```python
from build123d import *

# Parameters (mm, degrees)
SKETCH_1_R               = 6
EXTRUDE_1_DEPTH          = 15
SKETCH_2_OUTSIDE_W       = 18.53
SKETCH_2_OUTSIDE_H       = 18.53
SKETCH_2_OUTSIDE_W_2     = 10
SKETCH_2_OUTSIDE_H_2     = 17.562426414
CUT_EXTRUDE_1_DEPTH      = 15
EXTRUDE_2_DEPTH          = 1
SKETCH_4_W               = 10
SKETCH_4_H               = 12
EXTRUDE_3_DEPTH          = 10
SKETCH_5_R               = 1.5
EXTRUDE_4_DEPTH          = 10
SKETCH_6_W               = 6.926984356
SKETCH_6_H               = 2.009610912
CUT_EXTRUDE_2_DEPTH      = 10
SKETCH_7_R               = 5
EXTRUDE_5_DEPTH          = 4
SKETCH_8_W               = 7.4
SKETCH_8_H               = 10
EXTRUDE_6_DEPTH          = 4
HOLE_WIZARD_M1_4_1_D     = 1.6
HOLE_WIZARD_M1_4_1_DEPTH = 10
HOLE_WIZARD_M1_4_1_TIP   = 0.480688495
HOLE_WIZARD_M1_6_1_D     = 1.25
HOLE_WIZARD_M1_6_1_DEPTH = 4
HOLE_WIZARD_M1_6_1_TIP   = 0.375537887


with BuildPart() as part:
    # 草图1 → 凸台-拉伸1 (new body)
    with BuildSketch(Plane(origin=(0, 0, 0), x_dir=(1, 0, 0), z_dir=(0, 1, 0))):
        with Locations(Location((0, 0, 0), (0, 0, 270))):
            Circle(SKETCH_1_R)
    extrude(amount=EXTRUDE_1_DEPTH)

    # 草图2 outside → 切除-拉伸1 (cut)
    with BuildSketch(Plane(origin=(0, 15, 0), x_dir=(1, 0, 0), z_dir=(0, 1, 0))):
        Rectangle(SKETCH_2_OUTSIDE_W, SKETCH_2_OUTSIDE_H)
        Rectangle(SKETCH_2_OUTSIDE_W_2, SKETCH_2_OUTSIDE_H_2, mode=Mode.SUBTRACT)
    extrude(amount=-CUT_EXTRUDE_1_DEPTH, mode=Mode.SUBTRACT)

    # 草图3 → 凸台-拉伸2 (add)
    with BuildSketch(Plane(origin=(0, 15, 0), x_dir=(1, 0, 0), z_dir=(0, 1, 0))):
        with BuildLine():
            Line((0, -6), (-15, -6))
            Line((-15, -6), (-15, 6))
            Line((-15, 6), (0, 6))
            ThreePointArc((0, 6), (2.837274331, 5.286764074), (5, 3.31662479))
            Line((5, 3.31662479), (5, -3.31662479))
            ThreePointArc((5, -3.31662479), (2.837274331, -5.286764074), (0, -6))
        make_face()
    extrude(amount=EXTRUDE_2_DEPTH)

    # 草图4 → 凸台-拉伸3 (add)
    with BuildSketch(Plane.XZ):
        Rectangle(SKETCH_4_W, SKETCH_4_H)
    extrude(amount=EXTRUDE_3_DEPTH)

    # 草图5 → 凸台-拉伸4 (add)
    with BuildSketch(Plane.XZ.offset(10)):
        with Locations(Location((0, 0, 0), (0, 0, 270))):
            Circle(SKETCH_5_R)
    extrude(amount=EXTRUDE_4_DEPTH)

    # 草图6 → 切除-拉伸2 (cut)
    with BuildSketch(Plane.XZ.offset(20)):
        with Locations((0.466792476, -2.004805456)):
            Rectangle(SKETCH_6_W, SKETCH_6_H)
    extrude(amount=-CUT_EXTRUDE_2_DEPTH, mode=Mode.SUBTRACT)

    # 草图7 → 凸台-拉伸5 (add)
    with BuildSketch(Plane(origin=(0, 16, 0), x_dir=(1, 0, 0), z_dir=(0, 1, 0))):
        Circle(SKETCH_7_R)
    extrude(amount=EXTRUDE_5_DEPTH)

    # 草图8 → 凸台-拉伸6 (add)
    with BuildSketch(Plane(origin=(0, 16, 0), x_dir=(1, 0, 0), z_dir=(0, 1, 0))):
        with Locations((-13.7, 0)):
            Rectangle(SKETCH_8_W, SKETCH_8_H)
    extrude(amount=EXTRUDE_6_DEPTH)

    # M1.4 间隙孔1
    with Locations(Plane(origin=(0, -10, 0), x_dir=(-1, 0, 0), z_dir=(0, -1, 0))):
        with Locations((-2.5, 3.75), (2.5, -3.75)):
            Hole(HOLE_WIZARD_M1_4_1_D / 2, depth=HOLE_WIZARD_M1_4_1_DEPTH)
            with Locations((0, 0, -(HOLE_WIZARD_M1_4_1_DEPTH + HOLE_WIZARD_M1_4_1_TIP / 2))):  # 118° drill point
                Cone(0, HOLE_WIZARD_M1_4_1_D / 2, HOLE_WIZARD_M1_4_1_TIP, mode=Mode.SUBTRACT)

    # M1.6 螺纹孔1
    with Locations(Plane(origin=(0, -10, 0), x_dir=(-1, 0, 0), z_dir=(0, -1, 0))):
        with Locations((0, 5), (0, -5)):
            Hole(HOLE_WIZARD_M1_6_1_D / 2, depth=HOLE_WIZARD_M1_6_1_DEPTH)
            with Locations((0, 0, -(HOLE_WIZARD_M1_6_1_DEPTH + HOLE_WIZARD_M1_6_1_TIP / 2))):  # 118° drill point
                Cone(0, HOLE_WIZARD_M1_6_1_D / 2, HOLE_WIZARD_M1_6_1_TIP, mode=Mode.SUBTRACT)


solid = part.part
```
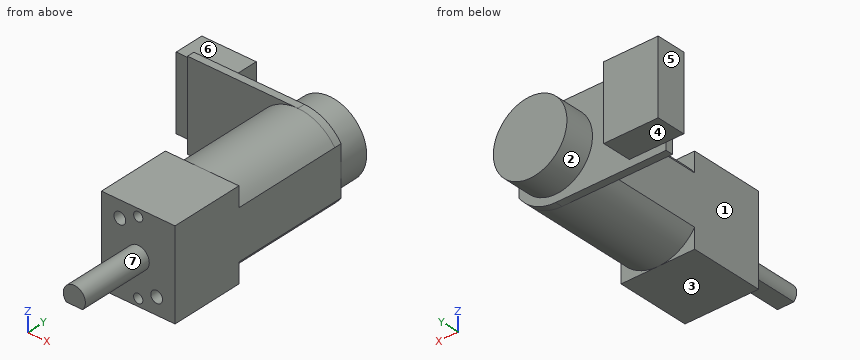
Part model, mm, in its own coordinate system. Face numbers are marked on the shaded views. A direction names the side the tool comes from. Round coordinates to 2 decimals unless told otherwise and drop trailing zeros. Order: outer loops, then holes, each group sorted by start corner. A loop starts at its lowest first (then second) coordinate and runs counter-clockwise, first axis right, second up. Notation, with made-up numbers: M -39.75,44 L 14.25,44 A20 cw 14.25,65 Z; hole C 22,7.5 d2. An arc over 180 degrees is marked long. Answer in a Markdown table with one row per item. Add a question column.
Q1. Cut at A-A on x = -13.5. Give the cut face in (y, z), and give its area (3 significant figures).
Q2. Mould opens along X. For the marked faces 1, 2 and 3 say: +X half, -X half, draft (parallel to the pull), parting line (faces both ways), or undercut.
Q3. Pin check, flat tips, straight feed: pin 1 (0.7 mm diameter, centred on x = -15.5, z = -1.5, fed in from -Y); pin 2 (1 mm diameter, centred on x = -6, y = -10, fed in from +Z); pin 3 (1 mm diameter, centred on y = 10.5, z = 2.5, fed in from -X); pin 4 (2 mm diameter, centred on x = -14.5, y = 17.5, fed in from +Z). Stop position of each tip, or through.
Q4. Cut at C-C on z = -2.25. Give the cut face in (x, y).
Q5. Cut at B-B on y = 13.5. Give the cut face in (x, z), and give its area (3 significant figures).
Q6. Wall check: L1, parallel to Z at x = 0, y = -8.1 (3 decimals); L2, parallel to X at y = -6.5, z = 3.75; L3, parallel to X at y = -8.6, z = -5 (3 decimals). Give the ranges that are in metal, low to high. Write a range as from..to.
Q7. 3-axis set-ups, long thin cutter, end or side, ignore diameter. For the marked faces 4, 5, 6 and 7: which of +Z, -Z, +X, -X, +Y, -Y reach the whole face in a straight line?
Q8. Cut at D-D on x = -8.5. Give the cut face in (y, z).
Established:
| question | item | result |
|---|---|---|
| 1 | outline | M 15,-6 L 16,-6 L 16,-5 L 20,-5 L 20,5 L 16,5 L 16,6 L 15,6 Z |
| 1 | area | 52.0 mm2 |
| 2 | face 1 | -X half |
| 2 | face 2 | undercut |
| 2 | face 3 | draft |
| 3 | pin 1 | stops at y = 16 |
| 3 | pin 2 | passes through |
| 3 | pin 3 | stops at x = -5 |
| 3 | pin 4 | stops at z = 5 |
| 4 | outline | M -17.4,16 L -15,16 L -15,15 L -5,15 L -5,-10 L 5,-10 L 5,16 L 4.47,16 L 4.47,20 L -4.47,20 L -4.47,16 L -10,16 L -10,20 L -17.4,20 Z |
| 5 | outline | M -5,-3.32 A6 ccw 5,-3.32 L 5,3.32 A6 ccw -5,3.32 Z |
| 5 | area | 104 mm2 |
| 6 | L1 | z = -6..-5.625, -4.375..4.375, 5.625..6 |
| 6 | L2 | x = -5..-3.3, -1.7..5 |
| 6 | L3 | x = -5..-0.625, 0.625..5 |
| 7 | face 4 | -Z, +X, -X, +Y |
| 7 | face 5 | +Z, -Z, -X, +Y, -Y |
| 7 | face 6 | +Z, +X, -X, +Y |
| 7 | face 7 | -Y |
| 8 | outline | M 15,-6 L 16,-6 L 16,6 L 15,6 Z |
